Part model, mm, in its own coordinate system. Give positions to 0.01 mm unless a question says otherwise; leave off trailing zeros. Write each loop counter-clockwise with the first axis right and the second up, starting at its lowest first coordinate (ties: lowest second). Pieces come first, ordered by that corner, then holes.
from build123d import *

# Parameters (mm, degrees)
CROQUIS1_R              = 10
SALIENTE_EXTRUIR1_DEPTH = 8
REDONDEO1_R             = 1.5
CROQUIS3_R              = 1
CORTAR_EXTRUIR1_DEPTH   = 9


with BuildPart() as part:
    # Croquis1 → Saliente-Extruir1 (new body)
    with BuildSketch(Plane.XY):
        Circle(CROQUIS1_R)
    extrude(amount=SALIENTE_EXTRUIR1_DEPTH)

    # Redondeo1
    redondeo1_edges = [part.edges().sort_by_distance(p)[0] for p in [
        (-10, 0, 0),
        (-10, 0, 8),
    ]]
    fillet(redondeo1_edges, radius=REDONDEO1_R)

    # Croquis3 → Cortar-Extruir1 (cut, through all)
    with BuildSketch(Plane.XY.offset(8)):
        Circle(CROQUIS3_R)
    extrude(amount=-CORTAR_EXTRUIR1_DEPTH, mode=Mode.SUBTRACT)


solid = part.part
1) Flat gauge pins, fed straight in: P1, Ø2, axis at y = -6, z = 7, coming from the -X side; P2, Ø2, axis at y = -6.5, z = 5.5, coming from the +X side; P3, Ø1.5, axis at y = 6, z = 7, coming from the +X side. Where does each tip first touch, or does it go through?
Check result:
P1: stops at x = -8.62
P2: stops at x = 8.35
P3: stops at x = 8.46
2) Saw through at D-D (z = 1). Write the cut outline in (x, y), and give its area (3 significant figures).
Check result:
outline: circle Ø19.83 at (0, 0); hole circle Ø2 at (0, 0)
area: 306 mm2
3) Saw through at C-C (z = 4). Write the cut outline in (x, y).
Check result:
outline: circle Ø20 at (0, 0); hole circle Ø2 at (0, 0)
4) Drill centre lines: L1, parallel to Y at x = 0, z = 5.75; L2, parallel to X at y = 0.5, z = 6.25; L3, parallel to X at y = 0.5, z = 7.5. Where is each one in solid material? Low to high.
Check result:
L1: y = -10 to -1, 1 to 10
L2: x = -9.99 to -0.87, 0.87 to 9.99
L3: x = -9.61 to -0.87, 0.87 to 9.61
5) Saw through at A-A (y = 0). Write the cut outline in (x, z).
Check result:
outline: (-10, 1.5) arc R1.5 ccw to (-8.5, 0) - (-1, 0) - (-1, 8) - (-8.5, 8) arc R1.5 ccw to (-10, 6.5) - close; (1, 0) - (8.5, 0) arc R1.5 ccw to (10, 1.5) - (10, 6.5) arc R1.5 ccw to (8.5, 8) - (1, 8) - close
6) Mould opens along Y. For faces 1 (the cylindrical face through (0, -1, 4)), 2 (the cylindrical face through (-2.17, -9.76, 3.96)), 3 (the flat face through (2, 0, 8)) say: +Y half, -Y half, draft (parallel to the pull), parting line (faces both ways), or undercut.
Check result:
face 1: undercut
face 2: parting line
face 3: draft
